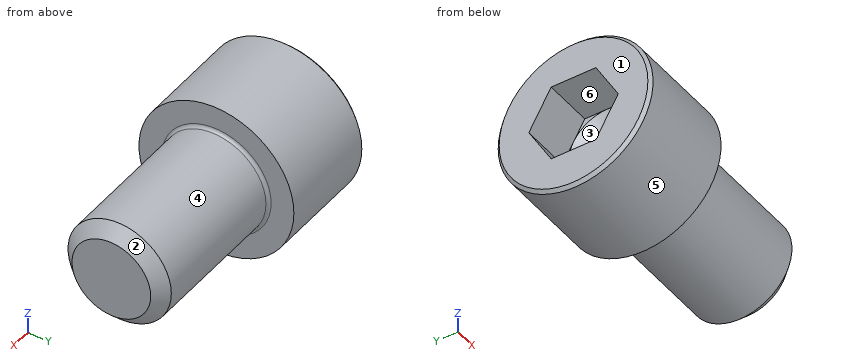
Autodesk Inventor part; units mm, degrees
ref_plane "screw_XY" through (0, 0, 0) normal (1, 0, 0) x (0, 0, -1)
ref_plane "screw_YZ" through (0, 0, 0) normal (0, 0, -1) x (0, 1, 0)
ref_plane "screw_ZX" through (0, 0, 0) normal (0, 1, 0) x (1, 0, 0)
sketch "Sketch_1" plane through (0, 0, 0) normal (0, 0, 1) x (1, 0, 0)
  line L0 (9.525, 0) -> (-6.35, 0)
  line L1 (-6.35, 0) -> (-6.35, 4.572)
  line L2 (-6.35, 4.572) -> (-6.1595, 4.7625)
  line L3 (-6.1595, 4.7625) -> (0, 4.7625)
  line L4 (0, 4.7625) -> (0, 3.3655)
  arc A0 (0, 3.3655) -> (0.1905, 3.175) centre (0.1905, 3.3655) ccw
  line L5 (0.1905, 3.175) -> (8.7693, 3.175)
  line L6 (8.7693, 3.175) -> (9.525, 2.4194)
  line L7 (9.525, 2.4194) -> (9.525, 0)
  line L8 (9.525, 0) -> (-6.35, 0)
revolve "Revolution1" add sketch "Sketch_1" angle 360 about axis through (9.525, 0, 0) along (1, 0, 0)
thread "Thread1"
sketch "Sketch_3" plane through (-6.35, 0, 0) normal (1, 0, 0) x (0, 0, -1)
  line L0 (-2.3813, -1.3748) -> (0, -2.7496)
  line L1 (0, -2.7496) -> (2.3813, -1.3748)
  line L2 (2.3813, -1.3748) -> (2.3813, 1.3748)
  line L3 (2.3813, 1.3748) -> (0, 2.7496)
  line L4 (0, 2.7496) -> (-2.3813, 1.3748)
  line L5 (-2.3813, 1.3748) -> (-2.3813, -1.3748)
extrude "Extrusion1" cut sketch "Sketch_3" along normal blind 3.048
sketch "Sketch_4" plane through (0, 0, 0) normal (0, 0, 1) x (1, 0, 0)
  line L0 (-1.9272, 0) -> (-3.302, 0)
  line L1 (-3.302, 0) -> (-3.302, 2.3813)
  line L2 (-3.302, 2.3813) -> (-1.9272, 0)
  line L3 (-1.9272, 0) -> (-3.302, 0)
revolve "Revolution2" cut sketch "Sketch_4" angle 360 about axis through (-1.9272, 0, 0) along (1, 0, 0)
ref_plane "screw_XY" through (0, 0, 0) normal (1, 0, 0) x (0, 0, -1)
ref_plane "screw_YZ" through (0, 0, 0) normal (0, 0, -1) x (0, 1, 0)
ref_plane "screw_ZX" through (0, 0, 0) normal (0, 1, 0) x (1, 0, 0)
ref_plane "screw1_XY" through (9.525, 0, 0) normal (1, 0, 0) x (0, 0, -1)
ref_plane "screw1_YZ" through (9.525, 0, 0) normal (0, 0, -1) x (0, 1, 0)
ref_plane "screw1_ZX" through (9.525, 0, 0) normal (0, 1, 0) x (1, 0, 0)
ref_plane "screw2_XY" through (4.445, 0, 0) normal (1, 0, 0) x (0, 0, -1)
ref_plane "screw2_YZ" through (4.445, 0, 0) normal (0, 0, -1) x (0, 1, 0)
ref_plane "screw2_ZX" through (4.445, 0, 0) normal (0, 1, 0) x (1, 0, 0)
ref_plane "to_tnut_XY" through (7.366, 0, 0) normal (1, 0, 0) x (0, 0, -1)
ref_plane "to_tnut_YZ" through (7.366, 0, 0) normal (0, 0, -1) x (0, 1, 0)
ref_plane "to_tnut_ZX" through (7.366, 0, 0) normal (0, 1, 0) x (1, 0, 0)
properties part number "3058"
Geometry: final body of the model. Coordinates: model frame, mm. Face numbers are marked on the shaded views. A direction names the side the tool comes from. Round coordinates to 2 decimals unless told otherwise and drop trailing zeros. Write each loop counter-clockwise with the first axis right and the second up, starting at its lowest first coordinate (ties: lowest second). Pieces come first, ordered by that corner, then holes. Notation, with made-up numbers: M 29.5,-6 L 73.5,-6 A10 ccw 73.5,1 Z; hole C 82.5,20 d6. An arc over 180 degrees is marked long. Answer in a Markdown table with one row per item. Add a question column.
(1) Cut plane C-C, the plane x = -1. Return the cut outline in (y, z) (1 decimal).
(2) Cut plane A-A, the plane x = 6. Return the cut outline in (y, z) (3 decimals), then the cut area to 3 significant figures.
(3) Draft query along Y for the marked faces 1, 2 and 3. Return one class per face: pulls with the +Y half, pulls with the -Y half, needs draft (parallel to the pull), parting line crosses it, or undercut.
(4) Contact query for flat-ended pins moving along their axis: pin 1 (1.5 mm diameter, centred on y = -0.5, z = 2, fed in from -X); pin 2 (0.6 mm diameter, centred on y = -1, z = -2, fed in from -X). Output: stop coordinate, or through.
(5) Cut plane B-B, the plane x = -3. Return the cut outline in (y, z) (1 decimal).
(6) Reachability of the marked faces 4, 5 and 6 from +Z, -Z, +X, -X, +Y, -Y: full face, straight path, thin tool, end or side. Return the list, or none.
(7) Ray query, L1, parallel to Z at x = -4.75, y = -1.5; L2, parallel to X at y = 4, z = 0.75; L3, parallel to X at y = -1.5, z = 1.25 (3 decimals). Return the intervals inside material, ascending.
Established:
| question | item | result |
|---|---|---|
| 1 | outline | C 0,0 d9.5 |
| 2 | outline | C 0,0 d6.35 |
| 2 | area | 31.7 mm² |
| 3 | face 1 | needs draft |
| 3 | face 2 | parting line crosses it |
| 3 | face 3 | undercut |
| 4 | pin 1 | x = -6.35 |
| 4 | pin 2 | x = -3.3 |
| 5 | outline | C 0,0 d9.5; hole C 0,0 d3.7 |
| 6 | face 4 | +X |
| 6 | face 5 | +X, -X |
| 6 | face 6 | -X |
| 7 | L1 | -4.52 to -2.16, 2.16 to 4.52 |
| 7 | L2 | -6.35 to 0 |
| 7 | L3 | -3.054 to 9.525 |
